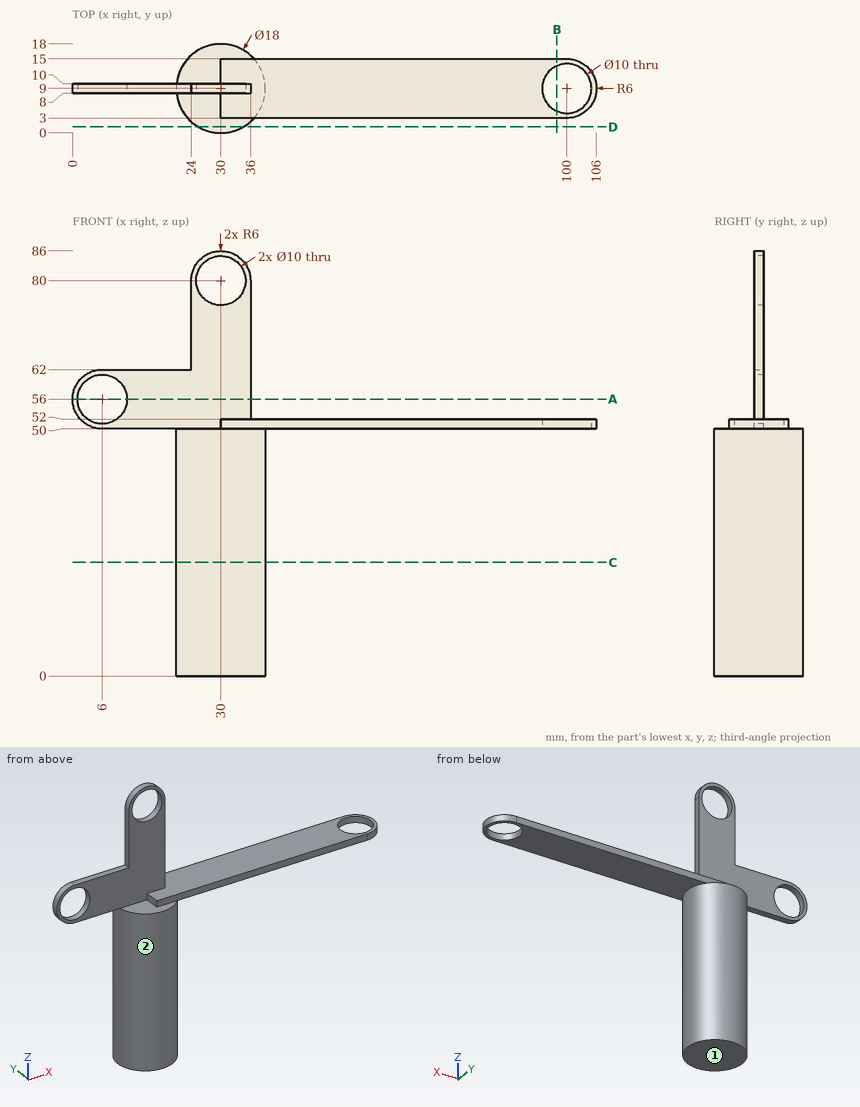
Here's the drawing with two shaded views (mm, measured from the low corner). I have some questions. A direction names the side the tool comes from. Round coordinates to 2 decimals unless told otherwise and drop trailing zeros. Loops run counter-clockwise (first coordinate to the right, second up) from the corner with the lowest first, then second, coordinate; pieces in that order, holes last.
Item 1: Which directions (+Z, -Z, +X, -X, +Y, -Y) give clear straight access to the entire face, cutting with the end or side of a thin tool? Please do the marked faces 1 and 2.
Item 2: Will these pins go through, and if not, where does the flat tip stop? pin 1 Ø1.6 at (x, z) = (79.5, 51) entering from +Y; pin 2 Ø9.5 at (x, y) = (63.5, 10) entering from +Z; pin 3 Ø6 at (x, y) = (79, 9) entering from -Z.
Item 3: Suppose I cut it at B-B, the plane x = 98. Write out the boundary of the cut face in (y, z).
Item 4: Please list where these lines run through material, in increasing order: L1, parallel to Z at x = 30, y = 8.65; L2, parallel to X at y = 9.4, z = 56; L3, parallel to Y at x = 30.5, z = 33.
Item 5: Suppose I cut it at A-A, the plane z = 56. Write out the boundary of the cut face in (x, y).
Item 6: Suppose I cut it at C-C, the plane z = 23. Write out the boundary of the cut face in (x, y).
Item 7: Suppose I cut it at D-D, the plane y = 1.25. Write out the boundary of the cut face in (x, z).
Reported:
1. face 1: -Z, +X, -X, +Y, -Y
1. face 2: -Z
2. pin 1: stops at y = 15
2. pin 2: stops at z = 52
2. pin 3: stops at z = 50
3. outline: (3, 50) - (4.42, 50) - (4.42, 52) - (3, 52) - close; (13.58, 50) - (15, 50) - (15, 52) - (13.58, 52) - close
4. L1: z = 0 to 75, 85 to 86
4. L2: x = 0 to 1, 11 to 36
4. L3: y = 0.01 to 17.99
5. outline: (0, 8) - (1, 8) - (1, 10) - (0, 10) - close; (11, 8) - (36, 8) - (36, 10) - (11, 10) - close
6. outline: circle Ø18 at (30, 9)
7. outline: (25.42, 0) - (34.58, 0) - (34.58, 50) - (25.42, 50) - close
